Drawing for the job (mm, zero at the part's lowest x, y, z). A direction names the side the tool comes from. Round coordinates to 2 decimals unless told otherwise and drop trailing zeros. Order: outer loops, then holes, each group sorted by start corner. A loop starts at its lowest first (then second) coordinate and runs counter-clockwise, first axis right, second up. Notation, with made-up numbers: (79.5, -32) - (99.5, -32) arc R22 cw to (99.5, 1) - close; hole circle Ø11 at (83, -19.5). An arc over 180 degrees is marked (long way). Answer as a JSON object with one key per item and string values.
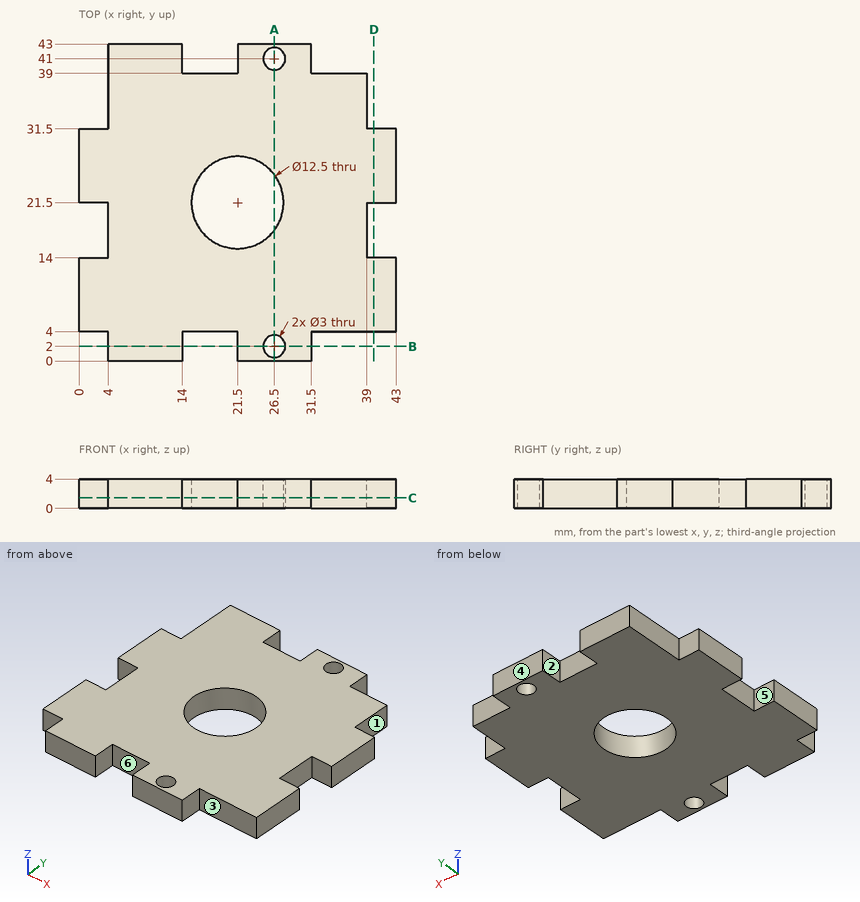
Item 1: Drop flat-ended pins along their axis: P1, Ø1.2, axis at x = 39, z = 1, coming from the -Y side; P2, Ø2, axis at x = 35, z = 2.5, coming from the +Y side; P3, Ø1.2, axis at y = 1.5, z = 2, coming from the +X side. Give the stop position or say it passes through.
Taken from the geometry:
{"P1": "y = 4", "P2": "y = 39", "P3": "x = 31.5"}
Item 2: Probe L1, parallel to Y at x = 26.5, z = 1.8; L2, parallel to X at y = 40.5, z = 1.7; L3, parallel to Y at x = 3, z = 1.5. List the from-to ranges inside material, lowest first. Write a range as from..to.
Taken from the geometry:
{"L1": "0..0.5, 3.5..17.75, 25.25..39.5, 42.5..43", "L2": "4..14, 21.5..25.09, 27.91..31.5", "L3": "4..14, 21.5..31.5"}
Item 3: Two-plate mould, pull along Y, no slides. Class the marked faces 4, 5 and 6: pulls with the +Y half, pulls with the -Y half, needs draft (parallel to the pull), parting line crosses it, or undercut.
Taken from the geometry:
{"face 4": "pulls with the +Y half", "face 5": "undercut", "face 6": "pulls with the -Y half"}
Item 4: Cut at D-D (x = 40). Write the cut outline in (y, z), plus the area to 3 significant figures.
Taken from the geometry:
{"outline": "(4, 0) - (14, 0) - (14, 4) - (4, 4) - close; (21.5, 0) - (31.5, 0) - (31.5, 4) - (21.5, 4) - close", "area": "80.0 mm2"}
Item 5: Cut at C-C (z = 1.45). State how many separate pieces and enclosed holes the cut face has, plus the area to 3 significant figures.
Taken from the geometry:
{"separate pieces": "1", "enclosed holes": "3", "area": "1,410 mm2"}
Item 6: Cut at A-A (x = 26.5). Write the cut outline in (y, z), plus the area to 3 significant figures.
Taken from the geometry:
{"outline": "(0, 0) - (0.5, 0) - (0.5, 4) - (0, 4) - close; (3.5, 0) - (17.75, 0) - (17.75, 4) - (3.5, 4) - close; (25.25, 0) - (39.5, 0) - (39.5, 4) - (25.25, 4) - close; (42.5, 0) - (43, 0) - (43, 4) - (42.5, 4) - close", "area": "118 mm2"}
Item 7: Cut at B-B (y = 2). Write the cut outline in (x, z), plus the area to 3 significant figures.
Taken from the geometry:
{"outline": "(4, 0) - (14, 0) - (14, 4) - (4, 4) - close; (21.5, 0) - (25, 0) - (25, 4) - (21.5, 4) - close; (28, 0) - (31.5, 0) - (31.5, 4) - (28, 4) - close", "area": "68.0 mm2"}
Item 8: Tool access for the marked faces 1, 2 and 3: list every direction of +Z, -Z, +X, -X, +Y, -Y with a clear straight run to the whole face (end or side of a thin tool).
Taken from the geometry:
{"face 1": "+Z, -Z, +X, +Y", "face 2": "+Z, -Z, +Y", "face 3": "+Z, -Z, +X, -Y"}
